For this review, take the finished solid that the model builds, in its own axes (mm). A direction names the side the tool comes from. Give positions to 0.01 mm unless a question says otherwise; leave off trailing zeros. Order: outer loops, then holes, each group sorted by start corner. A loop starts at its lowest first (then second) coordinate and runs counter-clockwise, first axis right, second up.
from build123d import *

# Parameters (mm, degrees)
SKETCH_1_W          = 102
SKETCH_1_H          = 70
EXTRUDE_1_DEPTH     = 5
SKETCH_2_W          = 85
SKETCH_2_H          = 56.6
CUT_EXTRUDE_1_DEPTH = 3.6
SKETCH_3_R          = 1
CUT_EXTRUDE_2_DEPTH = 6
SKETCH_5_W          = 100
SKETCH_5_H          = 68
CUT_EXTRUDE_4_DEPTH = 1
SKETCH_6_W          = 7
SKETCH_6_H          = 1
CUT_EXTRUDE_5_DEPTH = 1
SKETCH_7_W          = 65
SKETCH_7_H          = 36.6
CUT_EXTRUDE_6_DEPTH = 10
SKETCH_8_W          = 102
SKETCH_8_H          = 70
SKETCH_8_W_2        = 100
SKETCH_8_H_2        = 68
EXTRUDE_2_DEPTH     = 2


with BuildPart() as part:
    # Эскиз1 → Бобышка-Вытянуть1 (new body)
    with BuildSketch(Plane(origin=(0, 0, 0), x_dir=(1, 0, 0), z_dir=(0, 1, 0))):
        Rectangle(SKETCH_1_W, SKETCH_1_H)
    extrude(amount=EXTRUDE_1_DEPTH)

    # Эскиз2 → Вырез-Вытянуть1 (cut)
    with BuildSketch(Plane(origin=(0, 5, 0), x_dir=(1, 0, 0), z_dir=(0, 1, 0))):
        with Locations((-6.5, 0)):
            Rectangle(SKETCH_2_W, SKETCH_2_H)
    extrude(amount=-CUT_EXTRUDE_1_DEPTH, mode=Mode.SUBTRACT)

    # Эскиз3 → Вырез-Вытянуть2 (cut)
    with BuildSketch(Plane(origin=(0, 5, 0), x_dir=(1, 0, 0), z_dir=(0, 1, 0))):
        with Locations(Location((33, -31.5, 0), (0, 0, 270))):
            Circle(SKETCH_3_R)
        with Locations(Location((33, 31.5, 0), (0, 0, 270))):
            Circle(SKETCH_3_R)
        with Locations(Location((-46, -31.5, 0), (0, 0, 270))):
            Circle(SKETCH_3_R)
        with Locations(Location((-46, 31.5, 0), (0, 0, 270))):
            Circle(SKETCH_3_R)
    extrude(amount=-CUT_EXTRUDE_2_DEPTH, mode=Mode.SUBTRACT)

    # Эскиз5 → Вырез-Вытянуть4 (cut)
    with BuildSketch(Plane.XZ):
        Rectangle(SKETCH_5_W, SKETCH_5_H)
    extrude(amount=-CUT_EXTRUDE_4_DEPTH, mode=Mode.SUBTRACT)

    # Эскиз6 → Вырез-Вытянуть5 (cut)
    with BuildSketch(Plane.ZY.offset(51)):
        with Locations((0, 0.5)):
            Rectangle(SKETCH_6_W, SKETCH_6_H)
    extrude(amount=-CUT_EXTRUDE_5_DEPTH, mode=Mode.SUBTRACT)

    # Эскиз7 → Вырез-Вытянуть6 (cut)
    with BuildSketch(Plane(origin=(0, 1.4, 0), x_dir=(1, 0, 0), z_dir=(0, 1, 0))):
        with Locations((-6.5, 0)):
            Rectangle(SKETCH_7_W, SKETCH_7_H)
    extrude(amount=-CUT_EXTRUDE_6_DEPTH, mode=Mode.SUBTRACT)

    # Эскиз8 → Бобышка-Вытянуть2 (add)
    with BuildSketch(Plane(origin=(0, 5, 0), x_dir=(1, 0, 0), z_dir=(0, 1, 0))):
        Rectangle(SKETCH_8_W, SKETCH_8_H)
        Rectangle(SKETCH_8_W_2, SKETCH_8_H_2, mode=Mode.SUBTRACT)
    extrude(amount=EXTRUDE_2_DEPTH)


solid = part.part
1) Draft analysis for pull direction Z (two halves, no side actions). For faces 1 (the face through (-7, 3, -28.3)), 2 (the face through (51, 3, 0)), 3 (the face through (-1, 3, -35)), 4 (the face through (33.99, 3.03, -31.63)), state which applies: +Z half, -Z half, draft (parallel to the pull), parting line (faces both ways), or undercut.
Answer sheet:
face 1: undercut
face 2: draft
face 3: -Z half
face 4: undercut
2) To check wall thickness, follow line 1 (X direction, y = 2.1, z = 31.5); line 2 (Z direction, x = 1, y = 0.75); line 3 (Z direction, x = -5, y = 3.5). State the ranges of each line that lie inside material, in increasing order.
Answer sheet:
line 1: x = -51 to -47, -45 to 32, 34 to 51
line 2: z = -35 to -34, 34 to 35
line 3: z = -35 to -28.3, 28.3 to 35
3) We need section C-C on y = 3. Give the boundary of the cut face in (x, z).
Answer sheet:
outline: (-51, -35) - (51, -35) - (51, 35) - (-51, 35) - close; hole (-49, -28.3) - (36, -28.3) - (36, 28.3) - (-49, 28.3) - close; hole circle Ø2 at (-46, -31.5); hole circle Ø2 at (-46, 31.5); hole circle Ø2 at (33, -31.5); hole circle Ø2 at (33, 31.5)
4) We need section B-B on z = 14. Give the boundary of the cut face in (x, y), then the cut area to 3 significant figures.
Answer sheet:
outline: (-51, 0) - (-50, 0) - (-50, 1) - (-39, 1) - (-39, 1.4) - (-49, 1.4) - (-49, 5) - (-50, 5) - (-50, 7) - (-51, 7) - close; (26, 1) - (50, 1) - (50, 0) - (51, 0) - (51, 7) - (50, 7) - (50, 5) - (36, 5) - (36, 1.4) - (26, 1.4) - close
area: 82.0 mm2
5) Tool access review of faces 5 (the face through (-7, 3, 28.3)), 6 (the face through (-45.01, 3.03, -31.63)): name each direction out of +Z, -Z, +X, -X, +Y, -Y from which nothing blocks a thin tool from reaching the whole face with its end or side.
Answer sheet:
face 5: +Y
face 6: +Y, -Y
6) Clearance check with flat-ended pins moving along their axes: pin 1 (2.5 mm diameter, centred on x = 33, z = -31.5, fed in from +Y); pin 2 (1.6 mm diameter, centred on x = -46, z = 31.5, fed in from -Y); pin 3 (2.5 mm diameter, centred on x = 33, z = 31.5, fed in from -Y); pin 4 (20.5 mm diameter, centred on x = 2, z = -17, fed in from +Y). State where each tip first meets the part, or that it passes through.
Answer sheet:
pin 1: stops at y = 5
pin 2: passes through
pin 3: stops at y = 1
pin 4: stops at y = 1.4
7) We need section A-A on x = -20. Give the boundary of the cut face in (y, z), then the cut area to 3 significant figures.
Answer sheet:
outline: (0, -35) - (7, -35) - (7, -34) - (5, -34) - (5, -28.3) - (1.4, -28.3) - (1.4, -18.3) - (1, -18.3) - (1, -34) - (0, -34) - close; (0, 34) - (1, 34) - (1, 18.3) - (1.4, 18.3) - (1.4, 28.3) - (5, 28.3) - (5, 34) - (7, 34) - (7, 35) - (0, 35) - close
area: 67.6 mm2
8) We need section D-D on x = 33. Give the boundary of the cut face in (y, z).
Answer sheet:
outline: (0, -35) - (7, -35) - (7, -34) - (5, -34) - (5, -32.5) - (1, -32.5) - (1, -34) - (0, -34) - close; (0, 34) - (1, 34) - (1, 32.5) - (5, 32.5) - (5, 34) - (7, 34) - (7, 35) - (0, 35) - close; (1, -30.5) - (5, -30.5) - (5, -28.3) - (1.4, -28.3) - (1.4, 28.3) - (5, 28.3) - (5, 30.5) - (1, 30.5) - close
